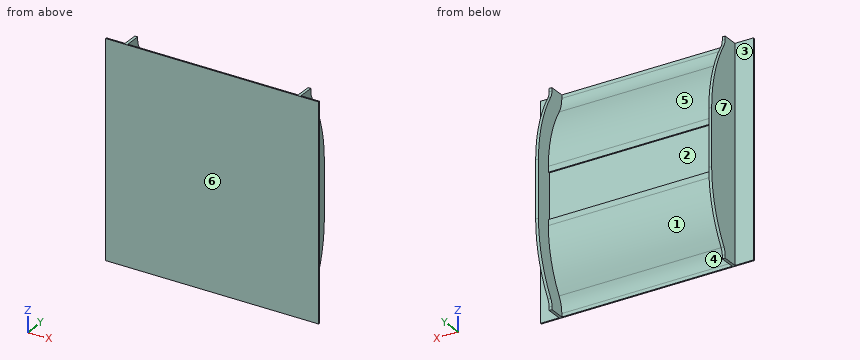
from build123d import *

# Parameters (mm, degrees)
SKETCH2_W           = 1500
SKETCH2_H           = 1500
BOSS_EXTRUDE1_DEPTH = 10
BOSS_EXTRUDE3_DEPTH = 1240
BOSS_EXTRUDE4_DEPTH = 20
SKETCH6_W           = 1200
SKETCH6_H           = 320
CUT_EXTRUDE1_DEPTH  = 10


with BuildPart() as part:
    # Sketch2 → Boss-Extrude1 (new body)
    with BuildSketch(Plane(origin=(0, 0, 0), x_dir=(1, 0, 0), z_dir=(0, 1, 0))):
        Rectangle(SKETCH2_W, SKETCH2_H)
    extrude(amount=BOSS_EXTRUDE1_DEPTH)

    # Sketch4 → Boss-Extrude3 (add)
    with BuildSketch(Plane.ZY.offset(620)):
        with BuildLine():
            ThreePointArc((-621.426146358, 40.000002328), (-672.010429767, 17.646159988), (-726.782687643, 10))
            Line((-726.782687643, 10), (726.782687643, 10))
            ThreePointArc((726.782687643, 10), (672.010424989, 17.646161349), (621.426137912, 40.000007562))
            ThreePointArc((621.426137912, 40.000007562), (419.089016099, 129.415364432), (200, 160))
            Line((200, 160), (-200, 160))
            ThreePointArc((-200, 160), (-419.089020877, 129.415363072), (-621.426146358, 40.000002328))
        make_face()
    extrude(amount=-BOSS_EXTRUDE3_DEPTH)

    # Sketch5 → Boss-Extrude4 (add)
    with BuildSketch(Plane.ZY.offset(620)):
        with BuildLine():
            Line((-750, 120), (-750, 10))
            Line((-750, 10), (-726.782687643, 10))
            ThreePointArc((-726.782687643, 10), (-672.010429767, 17.646159988), (-621.426146358, 40.000002328))
            ThreePointArc((-621.426146358, 40.000002328), (-419.089020877, 129.415363072), (-200, 160))
            Line((-200, 160), (200, 160))
            ThreePointArc((200, 160), (419.089016099, 129.415364432), (621.426137912, 40.000007562))
            ThreePointArc((621.426137912, 40.000007562), (672.010424989, 17.646161349), (726.782687643, 10))
            Line((726.782687643, 10), (750, 10))
            Line((750, 10), (750, 120))
            Line((750, 120), (726.782687643, 120))
            ThreePointArc((726.782687643, 120), (702.135172555, 123.440771722), (679.372245755, 133.5))
            ThreePointArc((679.372245755, 133.5), (449.213763665, 235.209974806), (200, 270))
            Line((200, 270), (-200, 270))
            ThreePointArc((-200, 270), (-449.213763665, 235.209974806), (-679.372245755, 133.5))
            ThreePointArc((-679.372245755, 133.5), (-702.135172555, 123.440771722), (-726.782687643, 120))
            Line((-726.782687643, 120), (-750, 120))
        make_face()
    boss_extrude4 = extrude(amount=-BOSS_EXTRUDE4_DEPTH)

    # Mirror1: Boss-Extrude4 across plane
    add(boss_extrude4.mirror(Plane(origin=(0, 0, 0), x_dir=(0, 0, 1), z_dir=(1, 0, 0))))

    # Sketch6 → Cut-Extrude1 (cut)
    with BuildSketch(Plane(origin=(0, 160, 0), x_dir=(1, 0, 0), z_dir=(0, 1, 0))):
        Rectangle(SKETCH6_W, SKETCH6_H)
    extrude(amount=-CUT_EXTRUDE1_DEPTH, mode=Mode.SUBTRACT)


solid = part.part
Here's how the part is built. I have some questions about the finished solid (model axes, mm). Face numbers are marked on the shaded views. A direction names the side the tool comes from. Give positions to 0.01 mm unless a question says otherwise; leave off trailing zeros. Order: outer loops, then holes, each group sorted by start corner. A loop starts at its lowest first (then second) coordinate and runs counter-clockwise, first axis right, second up. Notation, with made-up numbers: (51.25, 6.25) -> (56.25, 6.25) arc R18 cw to (56.25, 41.25) -> close; hole circle Ø7 at (89.5, 51.25). An arc over 180 degrees is marked (long way). One line per item, written item: value. Start each with the question number.
1. Imagine slicing it at C-C, the plane z = -318. List the corners of the cut face in (x, y) for me.
2. Imagine slicing it at D-D, the plane z = 355. List the corners of the cut face in (x, y) for me, plus the area to 3 significant figures.
3. Imagine slicing it at A-A, the plane y = 191. List the corners of the cut face in (x, z) for me.
4. For the marked faces 1, 2 and 3, which set-ups out of +Z, -Z, +X, -X, +Y, -Y let a thin tool reach every point of the face, with its end or its side?
5. I need wall thicknesses on probe 1 along X at (y, z) = (213.5, -87.5); probe 2 along Y at (x, z) = (513, -135.5); probe 3 along Y at (x, z) = (673, -520). Which ranges of each line are inside material? Lowest first, please. Write a range as from..to.
6. Imagine slicing it at B-B, the plane x = 566. List the corners of the cut face in (y, z) for me, plus the area to 3 significant figures.
7. Will these pins go through, and if not, where does the flat tip stop? pin 1 Ø1 at (y, z) = (206.5, 154) entering from +X; pin 2 Ø10 at (x, z) = (-612, -736.5) entering from +Y; pin 3 Ø18.5 at (x, z) = (-48.5, 737.5) entering from +Y.
8. We'd pull the mould along X, two halves only. Please class the marked faces 4, 5, 6 and 7: released by +X, released by -X, zero draft, split by the parting line, or undercut.
Values follow:
1. outline: (-750, 0) -> (750, 0) -> (750, 10) -> (620, 10) -> (620, 262.32) -> (600, 262.32) -> (600, 151.25) -> (-600, 151.25) -> (-600, 262.32) -> (-620, 262.32) -> (-620, 10) -> (-750, 10) -> close
2. outline: (-750, 0) -> (750, 0) -> (750, 10) -> (620, 10) -> (620, 256.7) -> (600, 256.7) -> (600, 144.84) -> (-600, 144.84) -> (-600, 256.7) -> (-620, 256.7) -> (-620, 10) -> (-750, 10) -> close
2. area: 187,000 mm2
3. outline: (-620, -570.86) -> (-600, -570.86) -> (-600, 570.86) -> (-620, 570.86) -> close; (600, -570.86) -> (620, -570.86) -> (620, 570.86) -> (600, 570.86) -> close
4. face 1: -Z, +Y
4. face 2: +Y
4. face 3: +Z, -Z, -X, +Y
5. probe 1: x = -620..-600, 600..620
5. probe 2: y = 0..150
5. probe 3: y = 0..10
6. outline: (0, -750) -> (10, -750) -> (10, -726.78) arc R200 cw to (40, -621.43) arc R800 ccw to (160, -200) -> (160, -160) -> (150, -160) -> (150, 160) -> (160, 160) -> (160, 200) arc R800 ccw to (40, 621.43) arc R200 cw to (10, 726.78) -> (10, 750) -> (0, 750) -> close
6. area: 168,000 mm2
7. pin 1: stops at x = 620
7. pin 2: stops at y = 120
7. pin 3: stops at y = 10
8. face 4: undercut
8. face 5: undercut
8. face 6: zero draft
8. face 7: released by -X
